from build123d import *

# Parameters (mm, degrees)
BOSS_EXTRUDE1_DEPTH = 3.175
SKETCH4_R           = 1.6
CUT_EXTRUDE3_DEPTH  = 153.126359575


with BuildPart() as part:
    # Sketch1 → Boss-Extrude1 (new, symmetric)
    with BuildSketch(Plane.XY):
        with BuildLine():
            Line((88.904443084, -50), (96.911769633, -50))
            ThreePointArc((96.911769633, -50), (-12.794056242, -108.31825077), (-105.853672586, -26))
            Line((-105.853672586, -26), (-98.630624048, -26))
            ThreePointArc((-98.630624048, -26), (-12.947959261, -101.174850388), (88.904443084, -50))
        make_face()
    extrude(amount=BOSS_EXTRUDE1_DEPTH, both=True)

    # Sketch4 → Cut-Extrude3 (cut, through all)
    with BuildSketch(Plane.XY.offset(3.175)):
        with Locations((-103.194571877, -21.934683381)):
            Circle(SKETCH4_R)
        with Locations((-105.407458575, -4.417881468)):
            Circle(SKETCH4_R)
        with Locations((-104.668100989, -13.222656141)):
            Circle(SKETCH4_R)
        with Locations((-100.336462469, 32.601292907)):
            Circle(SKETCH4_R)
        with Locations((104.295371407, 15.897342642)):
            Circle(SKETCH4_R)
        with Locations((100.708995202, 31.43164465)):
            Circle(SKETCH4_R)
        with Locations((94.822771885, 46.248155986)):
            Circle(SKETCH4_R)
        with Locations((-103.194571877, 21.934683381)):
            Circle(SKETCH4_R)
        with Locations((-104.668100989, 13.222656141)):
            Circle(SKETCH4_R)
        with Locations((-105.407458575, 4.417881468)):
            Circle(SKETCH4_R)
        with Locations((89.469074145, -55.906482377)):
            Circle(SKETCH4_R)
        with Locations((-44.130594647, 95.826617472)):
            Circle(SKETCH4_R)
        with Locations((-62.82106423, 84.757087545)):
            Circle(SKETCH4_R)
        with Locations((-78.848228037, 70.094271773)):
            Circle(SKETCH4_R)
        with Locations((-91.532612735, 52.45980181)):
            Circle(SKETCH4_R)
        with Locations((94.822771885, -46.248155986)):
            Circle(SKETCH4_R)
        with Locations((100.708995202, -31.43164465)):
            Circle(SKETCH4_R)
        with Locations((104.295371407, -15.897342642)):
            Circle(SKETCH4_R)
        with Locations((105.5, 0)):
            Circle(SKETCH4_R)
        with Locations((76.122528254, -73.04526468)):
            Circle(SKETCH4_R)
        with Locations((89.469074145, 55.906482377)):
            Circle(SKETCH4_R)
        with Locations((76.122528254, 73.04526468)):
            Circle(SKETCH4_R)
        with Locations((59.54875959, 87.08728513)):
            Circle(SKETCH4_R)
        with Locations((40.450414858, 97.437230758)):
            Circle(SKETCH4_R)
        with Locations((19.637170436, 103.656314507)):
            Circle(SKETCH4_R)
        with Locations((-2.008593938, 105.480877653)):
            Circle(SKETCH4_R)
        with Locations((-23.569203757, 102.833567643)):
            Circle(SKETCH4_R)
        with Locations((-91.532612735, -52.45980181)):
            Circle(SKETCH4_R)
        with Locations((-62.82106423, -84.757087545)):
            Circle(SKETCH4_R)
        with Locations((-44.130594647, -95.826617472)):
            Circle(SKETCH4_R)
        with Locations((-23.569203757, -102.833567643)):
            Circle(SKETCH4_R)
        with Locations((-2.008593938, -105.480877653)):
            Circle(SKETCH4_R)
        with Locations((19.637170436, -103.656314507)):
            Circle(SKETCH4_R)
        with Locations((40.450414858, -97.437230758)):
            Circle(SKETCH4_R)
        with Locations((59.54875959, -87.08728513)):
            Circle(SKETCH4_R)
        with Locations((-78.848228037, -70.094271773)):
            Circle(SKETCH4_R)
        with Locations((-100.336462469, -32.601292907)):
            Circle(SKETCH4_R)
    extrude(amount=-CUT_EXTRUDE3_DEPTH, mode=Mode.SUBTRACT)


solid = part.part
Read the model definition and answer for the solid it produces. Units are mm, in the model's axes. A direction names the side the tool comes from. Give positions to 0.01 mm unless a question says otherwise; leave off trailing zeros. Loops run counter-clockwise (first coordinate to the right, second up) from the corner with the lowest first, then second, coordinate; pieces in that order, holes last. Notation, with made-up numbers: (5.25, 56.25) -> (56.25, 56.25) arc R32 cw to (56.25, 83.25) -> close; hole circle Ø1 at (25.5, 32). An arc over 180 degrees is marked (long way). Use a Markdown table: item, result.
Q1. Find the intervals of material crossed by line 1 along X through (y, z) = (-57, -1.5); line 2 along X through (y, z) = (-70, -2); line 3 along X through (y, z) = (-89, 0.5), in increasing order.
Solved:
| item | result |
|---|---|
| line 1 | x = -92.94 to -84.59, 84.59 to 88.3, 90.64 to 92.97 |
| line 2 | x = -83.6 to -80.45, -77.25 to -74.19, 74.19 to 83.63 |
| line 3 | x = -63.01 to -49.83, 49.83 to 63.05 |
Q2. Determine the mould class of faces 3 (the face through (-10.95, -108.52, 0.04)), 4 (the face through (-14.626, -100.946, 0.044)), 5 (the face through (-102, -26, 0)) for opening direction X: pulls with the +X half, pulls with the -X half, needs draft (parallel to the pull), parting line crosses it, or undercut.
Solved:
| item | result |
|---|---|
| face 3 | parting line crosses it |
| face 4 | undercut |
| face 5 | needs draft |
Q3. Each of these flat-tipped pins is pushed along its axis until it touches: pin 1 (4 mm diameter, centred on x = 76.12, y = -73.05, fed in from +Z) (3 decimals); pin 2 (1 mm diameter, centred on y = -97.5, z = 1.5, fed in from +X); pin 3 (1.9 mm diameter, centred on x = -44.13, y = -95.83, fed in from +Z); pin 4 (3 mm diameter, centred on x = 94.5, z = -1, fed in from +Y). Where does it stop, or does it pass through?
Solved:
| item | result |
|---|---|
| pin 1 | stops at z = 3.175 |
| pin 2 | stops at x = 49.88 |
| pin 3 | passes through |
| pin 4 | stops at y = -50 |
Q4. Section A-A, the plane y = -77.5 is taken. Determine the outline of the cut face in (x, z) (3 decimals).
Solved:
| item | result |
|---|---|
| outline | (-76.703, -3.175) -> (-66.316, -3.175) -> (-66.316, 3.175) -> (-76.703, 3.175) -> close; (66.316, -3.175) -> (76.74, -3.175) -> (76.74, 3.175) -> (66.316, 3.175) -> close |
Q5. Section D-D, the plane x = -11 is taken. Determine the outline of the cut face in (y, z) (3 decimals), then the cut area to 3 significant figures.
Solved:
| item | result |
|---|---|
| outline | (-108.516, -3.175) -> (-101.405, -3.175) -> (-101.405, 3.175) -> (-108.516, 3.175) -> close |
| area | 45.2 mm^2 |
Q6. Section B-B, the plane z = -1.25 is taken. Count the separate pieces of the cut face and the enclosed holes in it, then the cut area to 3 significant figures.
Solved:
| item | result |
|---|---|
| separate pieces | 1 |
| enclosed holes | 12 |
| area | 1,690 mm^2 |
Q7. Section C-C, the plane y = -66 is taken. Determine the outline of the cut face in (x, z) (3 decimals), then the cut area to 3 significant figures.
Solved:
| item | result |
|---|---|
| outline | (-86.785, -3.175) -> (-77.769, -3.175) -> (-77.769, 3.175) -> (-86.785, 3.175) -> close; (77.769, -3.175) -> (86.821, -3.175) -> (86.821, 3.175) -> (77.769, 3.175) -> close |
| area | 115 mm^2 |
Q8. A tool of negligible diameter and unlimited length cuts with its end or side. For faces 1 (the face through (93, -50, 0)), 2 (the face through (-19, -101, 3.175)), from which of +Z, -Z, +X, -X, +Y, -Y can it reach the whole face along a straight path? Write none if from no direction.
Solved:
| item | result |
|---|---|
| face 1 | +Z, -Z, +X, +Y |
| face 2 | +Z, +X, -X, +Y, -Y |
